from build123d import *

# Parameters (mm, degrees)
CROQUIS1_W                   = 200
CROQUIS1_H                   = 200
CROQUIS1_R                   = 4.1
SALIENTE_EXTRUIR1_DEPTH      = 3
SALIENTE_EXTRUIR2_DEPTH      = 39
SALIENTE_EXTRUIR2_DEPTH_BACK = 3
SALIENTE_EXTRUIR3_DEPTH      = 5
REDONDEO1_R                  = 5
CROQUIS5_W                   = 100
CROQUIS5_H                   = 42
CORTAR_EXTRUIR2_DEPTH        = 12
CROQUIS6_R                   = 10
CORTAR_EXTRUIR3_DEPTH        = 10
CROQUIS7_R                   = 14
CORTAR_EXTRUIR4_DEPTH        = 4
REDONDEO2_R                  = 2
CROQUIS8_R                   = 10
CORTAR_EXTRUIR5_DEPTH        = 10
CROQUIS9_R                   = 14
CORTAR_EXTRUIR6_DEPTH        = 4
REDONDEO3_R                  = 2
CROQUIS11_W                  = 25.2
CROQUIS11_H                  = 16.7
CORTAR_EXTRUIR8_DEPTH        = 5
CROQUIS12_W                  = 25.2
CROQUIS12_H                  = 16.7
CORTAR_EXTRUIR9_DEPTH        = 5


with BuildPart() as part:
    # Croquis1 → Saliente-Extruir1 (new body)
    with BuildSketch(Plane(origin=(0, 0, 0), x_dir=(0, 1, 0), z_dir=(0, 0, 1))):
        Rectangle(CROQUIS1_W, CROQUIS1_H)
        with Locations(Location((-92.5, 92.5, 0), (0, 0, 270))):
            Circle(CROQUIS1_R, mode=Mode.SUBTRACT)
        with Locations(Location((92.5, 92.5, 0), (0, 0, 90))):
            Circle(CROQUIS1_R, mode=Mode.SUBTRACT)
        with Locations(Location((92.5, -92.5, 0), (0, 0, 270))):
            Circle(CROQUIS1_R, mode=Mode.SUBTRACT)
        with Locations(Location((-92.5, -92.5, 0), (0, 0, 90))):
            Circle(CROQUIS1_R, mode=Mode.SUBTRACT)
        Polygon((-95, 85), (-85, 85), (-85, 95), (85, 95), (85, 85), (95, 85), (95, -85), (85, -85), (85, -95), (-85, -95), (-85, -85), (-95, -85), align=None, mode=Mode.SUBTRACT)
    extrude(amount=SALIENTE_EXTRUIR1_DEPTH)

    # Croquis2 → Saliente-Extruir2 (add, two sides: drawn at the far end of the back side and taken through both)
    with BuildSketch(Plane.XY.offset(3).offset(-SALIENTE_EXTRUIR2_DEPTH_BACK)):
        Polygon((85, -85), (85, -95), (-85, -95), (-85, -85), (-95, -85), (-95, 85), (-85, 85), (-85, 95), (85, 95), (85, 85), (95, 85), (95, -85), align=None)
        Polygon((80, 90), (-80, 90), (-80, 80), (-90, 80), (-90, -80), (-80, -80), (-80, -90), (80, -90), (80, -80), (90, -80), (90, 80), (80, 80), align=None, mode=Mode.SUBTRACT)
    extrude(amount=SALIENTE_EXTRUIR2_DEPTH + SALIENTE_EXTRUIR2_DEPTH_BACK)

    # Croquis3 → Saliente-Extruir3 (add)
    with BuildSketch(Plane.XY.offset(42)):
        Polygon((85, -95), (85, -85), (95, -85), (95, 85), (85, 85), (85, 95), (-85, 95), (-85, 85), (-95, 85), (-95, -85), (-85, -85), (-85, -95), align=None)
        with BuildLine():
            Line((-58.921212306, 73.686200925), (-2.716957181, 73.686200925))
            ThreePointArc((-2.716957181, 73.686200925), (0.818576725, 72.221734831), (2.283042819, 68.686200925))
            Line((2.283042819, 68.686200925), (2.283042819, -9.052528374))
            ThreePointArc((2.283042819, -9.052528374), (0.818576725, -12.58806228), (-2.716957181, -14.052528374))
            Line((-2.716957181, -14.052528374), (-58.921212306, -14.052528374))
            ThreePointArc((-58.921212306, -14.052528374), (-62.456746212, -12.58806228), (-63.921212306, -9.052528374))
            Line((-63.921212306, -9.052528374), (-63.921212306, 68.686200925))
            ThreePointArc((-63.921212306, 68.686200925), (-62.456746212, 72.221734831), (-58.921212306, 73.686200925))
        make_face(mode=Mode.SUBTRACT)
    extrude(amount=SALIENTE_EXTRUIR3_DEPTH)

    # Redondeo1
    redondeo1_edges = [part.edges().sort_by_distance(p)[0] for p in [
        (-85, -85, 25),
        (-95, -85, 25),
        (-85, -95, 25),
        (95, -85, 25),
        (85, -85, 25),
        (85, -95, 25),
        (95, 85, 25),
        (85, 85, 25),
        (85, 95, 25),
        (-85, 85, 25),
        (-85, 95, 25),
        (-95, 85, 25),
        (100, 100, 1.5),
        (-100, 100, 1.5),
        (-100, -100, 1.5),
        (100, -100, 1.5),
        (-90, 80, 21),
        (-80, 80, 21),
        (-80, 90, 21),
        (80, 90, 21),
        (80, 80, 21),
        (90, 80, 21),
        (90, -80, 21),
        (80, -80, 21),
        (80, -90, 21),
        (-80, -90, 21),
        (-80, -80, 21),
        (-90, -80, 21),
    ]]
    fillet(redondeo1_edges, radius=REDONDEO1_R - 0.0001)  # a hair under: the kernel refuses the full size

    # Croquis5 → Cortar-Extruir2 (cut)
    with BuildSketch(Plane.XZ.offset(100)):
        with Locations((-25.139020419, 21)):
            Rectangle(CROQUIS5_W, CROQUIS5_H)
    extrude(amount=-CORTAR_EXTRUIR2_DEPTH, mode=Mode.SUBTRACT)

    # Croquis6 → Cortar-Extruir3 (cut)
    with BuildSketch(Plane.XZ.offset(95)):
        with Locations((52.430489791, 22.5)):
            Circle(CROQUIS6_R)
    extrude(amount=-CORTAR_EXTRUIR3_DEPTH, mode=Mode.SUBTRACT)

    # Croquis7 → Cortar-Extruir4 (cut)
    with BuildSketch(Plane(origin=(0, -90, 0), x_dir=(-1, 0, 0), z_dir=(0, 1, 0))):
        with Locations((-52.430489791, 22.5)):
            Circle(CROQUIS7_R)
    extrude(amount=-CORTAR_EXTRUIR4_DEPTH, mode=Mode.SUBTRACT)

    # Redondeo2
    redondeo2_edges = [part.edges().sort_by_distance(p)[0] for p in [
        (66.430489791, -90, 22.5),
    ]]
    fillet(redondeo2_edges, radius=REDONDEO2_R)

    # Croquis8 → Cortar-Extruir5 (cut)
    with BuildSketch(Plane(origin=(-95, 0, 0), x_dir=(0, -1, 0), z_dir=(-1, 0, 0))):
        with Locations((27.122609876, 22.5)):
            Circle(CROQUIS8_R)
    extrude(amount=-CORTAR_EXTRUIR5_DEPTH, mode=Mode.SUBTRACT)

    # Croquis9 → Cortar-Extruir6 (cut)
    with BuildSketch(Plane.YZ.offset(-90)):
        with Locations((-27.122609876, 22.5)):
            Circle(CROQUIS9_R)
    extrude(amount=-CORTAR_EXTRUIR6_DEPTH, mode=Mode.SUBTRACT)

    # Redondeo3
    redondeo3_edges = [part.edges().sort_by_distance(p)[0] for p in [
        (-90, -41.122609876, 22.5),
    ]]
    fillet(redondeo3_edges, radius=REDONDEO3_R)

    # Croquis11 → Cortar-Extruir8 (cut)
    with BuildSketch(Plane.XZ.offset(-95)):
        with Locations((22.4, 33.65)):
            Rectangle(CROQUIS11_W, CROQUIS11_H)
    extrude(amount=CORTAR_EXTRUIR8_DEPTH, mode=Mode.SUBTRACT)

    # Croquis12 → Cortar-Extruir9 (cut)
    with BuildSketch(Plane.YZ.offset(95)):
        with Locations((22.4, 33.65)):
            Rectangle(CROQUIS12_W, CROQUIS12_H)
    extrude(amount=-CORTAR_EXTRUIR9_DEPTH, mode=Mode.SUBTRACT)


solid = part.part
Can you work these out from the model? Positions are in its coordinate system, mm. A direction names the side the tool comes from. Coordinates: 2 decimals unless noted, no trailing zeros. Loops run counter-clockwise (first coordinate to the right, second up) from the corner with the lowest first, then second, coordinate; pieces in that order, holes last. Notation, with made-up numbers: M 29.5,29.25 L 85.5,29.25 A20 cw 85.5,67.25 Z; hole C 62.5,23.25 d7. An arc over 180 degrees is marked long. Answer as CSV lines item,"result". Start each with the question number.
1. Suppose I cut it at D-D, the plane y = 22.5. List the corners of the cut face in (x, z) for me.
2. Suppose I cut it at C-C, the plane x = 92.5. List the corners of the cut face in (y, z) for me, plus the area to 3 significant figures.
3. Thinking about a two-plate mould opening in Z: for faces 6 (the face through (45.97, -92.99, 10.08)), 7 (the face through (7, 96, 3)), 8 (the face through (-82, 81, 21)), which applies, +Z half, -Z half, draft (parallel to the pull), parting line (faces both ways), or undercut?
4. For faces 1 (the face through (-31, 73.686, 44)), 2 (the face through (94, -83, 25)), 3 (the face through (95, -1, 25)), 4 (the face through (22, 93, 25.3)), 5 (the face through (-90, 1, 21)), which set-ups out of +Z, -Z, +X, -X, +Y, -Y let a thin tool reach every point of the face, with its end or its side?
5. If I drill on probe 1 along Y at (x, z) = (-92.5, 1.35); probe 2 along Y at (x, z) = (40.5, 10), over which ranges is the centre line in solid material (lowest first)? Write a range as [from, to].
6. Suppose I cut it at A-A, the plane y = 56. List the corners of the cut face in (x, z) for me.
7. For pin 1 Ø8 at (y, z) = (-96, 25.5) entering from -X; pin 2 Ø1 at (y, z) = (10.5, 22) entering from +X; pin 3 Ø1.5 at (x, z) = (-24, 44.5) entering from +Y, each with a flat end and sliding along its axis, tell me the tip position at first contact or that it passes through.
Output:
1,outline,"M -100,0 L -90,0 L -90,42 L -63.92,42 L -63.92,47 L -95,47 L -95,3 L -100,3 Z; M 2.28,42 L 95,42 L 95,47 L 2.28,47 Z; M 90,0 L 100,0 L 100,3 L 95,3 L 95,25.3 L 90,25.3 Z"
2,outline,"M -100,0 L -96.6,0 L -96.6,3 L -100,3 Z; M -88.4,0 L 88.4,0 L 88.4,3 L 84.33,3 L 84.33,47 L -84.33,47 L -84.33,3 L -88.4,3 Z; M 96.6,0 L 100,0 L 100,3 L 96.6,3 Z; hole M 9.8,25.3 L 35,25.3 L 35,42 L 9.8,42 Z"
2,area,"7,550 mm^2"
3,face 6,"undercut"
3,face 7,"+Z half"
3,face 8,"draft"
4,face 1,"+Z, -Z"
4,face 2,"+Z, +X, -Y"
4,face 3,"+Z, +X, +Y, -Y"
4,face 4,"+Y"
4,face 5,"-Z"
5,probe 1,"y = [-100, -96.6], [-88.4, 88.4], [96.6, 100]"
5,probe 2,"y = [-95, -90], [90, 95]"
6,outline,"M -100,0 L -90,0 L -90,42 L -63.92,42 L -63.92,47 L -95,47 L -95,3 L -100,3 Z; M 2.28,42 L 90,42 L 90,0 L 100,0 L 100,3 L 95,3 L 95,47 L 2.28,47 Z"
7,pin 1,"stops at x = -84.58"
7,pin 2,"stops at x = 95"
7,pin 3,"stops at y = 95"
